Geometry: see drawing. Coordinates: mm, zero at the bounding-box minimum. A direction names the side the tool comes from. Round coordinates to 2 decimals unless told otherwise and drop trailing zeros. Loops run counter-clockwise (first coordinate to the right, second up) from the corner with the lowest first, then second, coordinate; pieces in that order, holes last. Notation, with made-up numbers: (-14, 76.5) - (1, 76.5) arc R23 ccw to (1, 107.5) - close; hole circle Ø1 at (72.5, 82). An arc over 180 degrees is marked (long way). Return JSON: item names as keys, results as strings. Group by question number.
1. Section B-B on x = 41.5. Return loops of the section in (y, z).
2. Section A-A on y = 13.5. Return loops of the section in (x, z).
3. First-contact query: pin 1 Ø4 at (x, z) = (3, 4) entering from +Y; pin 2 Ø19.5 at (y, z) = (13.5, 26) entering from -X; pin 3 Ø1.9 at (x, y) = (33, 36) entering from -Z. Flat tips, straight axial feed; report the tip coordinate or a pass-through.
4. Section D-D on z = 26. Return loops of the section in (x, y).
5. Section C-C on y = 41.5. Return loops of the section in (x, z).
6. Draft query along X for the marked faces 1, 2 and 3. Return one class per face: +X half, -X half, draft (parallel to the pull), parting line (faces both ways), or undercut.
7. Set-up query: the marked faces 4, 5, 6, 7 and 8. Return all of +Z, -Z, +X, -X, +Y, -Y with unobstructed straight access to the full face (end or side cutting, diameter ignored); none if empty.
8. Material intervals for probe 1 along Y at (x, z) = (33.5, 26); probe 2 along Y at (x, z) = (25.5, 27.5); probe 3 along Y at (x, z) = (3.75, 7.5), sorted ascending.
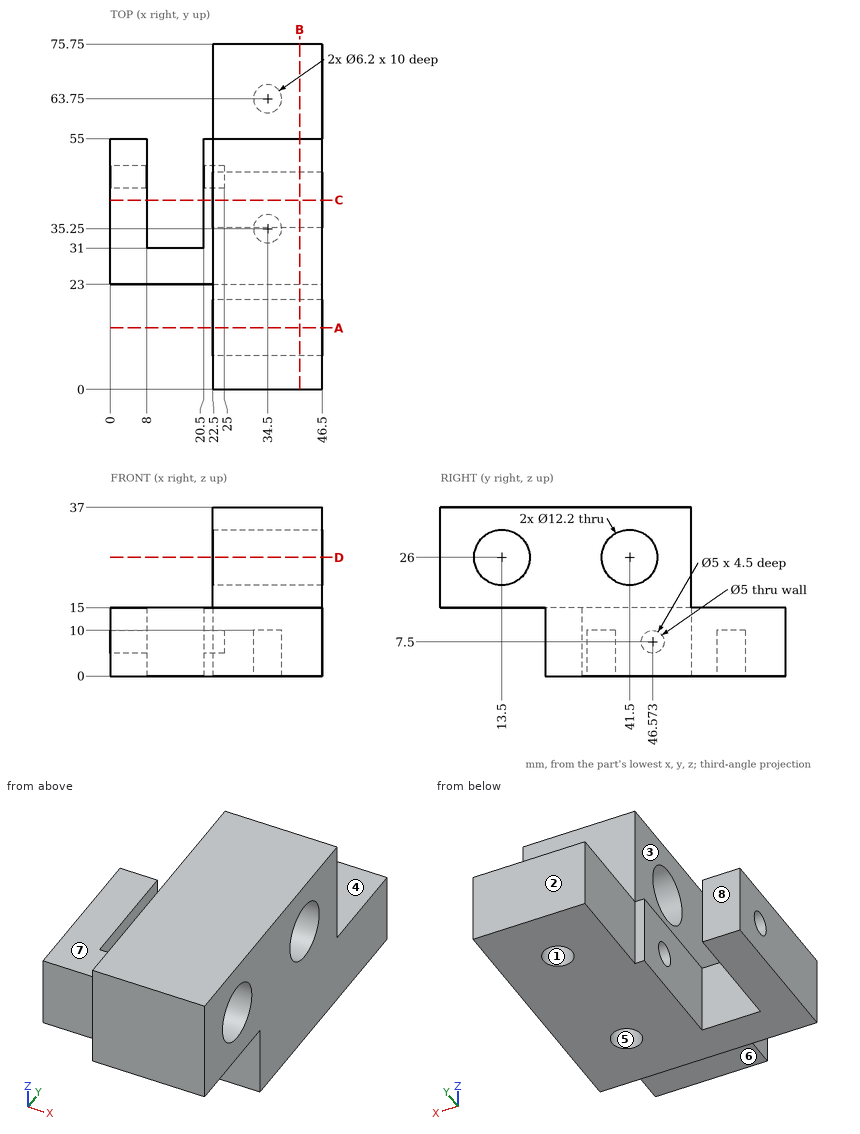
Taken from the geometry:
{
 "1": {"outline": "(0, 15) - (23, 15) - (23, 0) - (75.75, 0) - (75.75, 15) - (55, 15) - (55, 37) - (0, 37) - close; hole circle Ø12.2 at (13.5, 26); hole circle Ø12.2 at (41.5, 26)"},
 "2": {"outline": "(22.5, 15) - (46.5, 15) - (46.5, 19.9) - (22.5, 19.9) - close; (22.5, 32.1) - (46.5, 32.1) - (46.5, 37) - (22.5, 37) - close"},
 "3": {"pin 1": "y = 55", "pin 2": "x = 22.5", "pin 3": "z = 10"},
 "4": {"outline": "(22.5, 0) - (46.5, 0) - (46.5, 7.4) - (22.5, 7.4) - close; (22.5, 19.6) - (46.5, 19.6) - (46.5, 35.4) - (22.5, 35.4) - close; (22.5, 47.6) - (46.5, 47.6) - (46.5, 55) - (22.5, 55) - close"},
 "5": {"outline": "(0, 0) - (8, 0) - (8, 15) - (0, 15) - close; (20.5, 0) - (46.5, 0) - (46.5, 19.9) - (22.5, 19.9) - (22.5, 15) - (20.5, 15) - close; (22.5, 32.1) - (46.5, 32.1) - (46.5, 37) - (22.5, 37) - close"},
 "6": {"face 1": "undercut", "face 2": "draft", "face 3": "-X half"},
 "7": {"face 4": "+Z, +X, -X, +Y", "face 5": "-Z", "face 6": "-Z, +X, -X, -Y", "face 7": "+Z, -X, +Y, -Y", "face 8": "+Z, -Z, -X, +Y"},
 "8": {"probe 1": "0 to 7.4, 19.6 to 35.4, 47.6 to 55", "probe 2": "0 to 7.59, 19.41 to 35.59, 47.41 to 55", "probe 3": "23 to 44.07, 49.07 to 55"}
}
